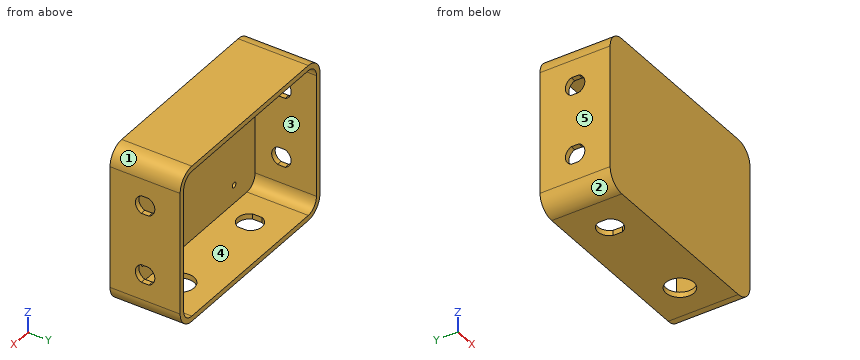
from build123d import *

# Parameters (mm, degrees)
BOSS_EXTRUDE1_DEPTH          = 5
F_3_0_3_DIAMETER_HOLE1_D     = 3
F_3_0_3_DIAMETER_HOLE1_DEPTH = 3
F_3_0_3_DIAMETER_HOLE1_TIP   = 0.901290929
BOSS_EXTRUDE2_DEPTH          = 35
CUT_EXTRUDE1_DEPTH           = 149
CUT_EXTRUDE2_DEPTH           = 35
SKETCH10_R                   = 8
CUT_EXTRUDE3_DEPTH           = 35


with BuildPart() as part:
    # Sketch1 → Boss-Extrude1 (new body)
    with BuildSketch(Plane(origin=(0, 0, 0), x_dir=(1, 0, 0), z_dir=(0, 1, 0))):
        with BuildLine():
            Line((10, 0), (110, 0))
            ThreePointArc((110, 0), (117.071067812, 2.928932188), (120, 10))
            Line((120, 10), (120, 80))
            ThreePointArc((120, 80), (117.071067812, 87.071067812), (110, 90))
            Line((110, 90), (10, 90))
            ThreePointArc((10, 90), (2.928932188, 87.071067812), (0, 80))
            Line((0, 80), (0, 10))
            ThreePointArc((0, 10), (2.928932188, 2.928932188), (10, 0))
        make_face()
    extrude(amount=BOSS_EXTRUDE1_DEPTH)

    # Ø3.0 (3) Diameter Hole1
    with Locations(Plane(origin=(0, 5, 0), x_dir=(1, 0, 0), z_dir=(0, 1, 0))):
        with Locations((99, 76.5), (21, 76.5), (21, 13.5), (99, 13.5)):
            Hole(F_3_0_3_DIAMETER_HOLE1_D / 2, depth=F_3_0_3_DIAMETER_HOLE1_DEPTH)
            with Locations((0, 0, -(F_3_0_3_DIAMETER_HOLE1_DEPTH + F_3_0_3_DIAMETER_HOLE1_TIP / 2))):  # 118° drill point
                Cone(0, F_3_0_3_DIAMETER_HOLE1_D / 2, F_3_0_3_DIAMETER_HOLE1_TIP, mode=Mode.SUBTRACT)

    # Sketch7 → Boss-Extrude2 (add)
    with BuildSketch(Plane(origin=(0, 5, 0), x_dir=(1, 0, 0), z_dir=(0, 1, 0))):
        with BuildLine():
            Line((10, 0), (110, 0))
            ThreePointArc((110, 0), (117.071067812, 2.928932188), (120, 10))
            Line((120, 10), (120, 80))
            ThreePointArc((120, 80), (117.071067812, 87.071067812), (110, 90))
            Line((110, 90), (10, 90))
            ThreePointArc((10, 90), (2.928932188, 87.071067812), (0, 80))
            Line((0, 80), (0, 10))
            ThreePointArc((0, 10), (2.928932188, 2.928932188), (10, 0))
        make_face()
        with BuildLine():
            Line((3, 80), (3, 10))
            ThreePointArc((3, 10), (5.050252532, 5.050252532), (10, 3))
            Line((10, 3), (110, 3))
            ThreePointArc((110, 3), (114.949747468, 5.050252532), (117, 10))
            Line((117, 10), (117, 80))
            ThreePointArc((117, 80), (114.949747468, 84.949747468), (110, 87))
            Line((110, 87), (10, 87))
            ThreePointArc((10, 87), (5.050252532, 84.949747468), (3, 80))
        make_face(mode=Mode.SUBTRACT)
    extrude(amount=BOSS_EXTRUDE2_DEPTH)

    # Sketch8 → Cut-Extrude1 (cut)
    with BuildSketch(Plane.ZY):
        with BuildLine():
            Line((-59.9, 22.189177928), (-59.9, 17.810822072))
            ThreePointArc((-59.9, 17.810822072), (-65, 14.45), (-70.1, 17.810822072))
            Line((-70.1, 17.810822072), (-70.1, 22.189177928))
            ThreePointArc((-70.1, 22.189177928), (-65, 25.55), (-59.9, 22.189177928))
        make_face()
        with BuildLine():
            Line((-19.9, 22.189177928), (-19.9, 17.810822072))
            ThreePointArc((-19.9, 17.810822072), (-25, 14.45), (-30.1, 17.810822072))
            Line((-30.1, 17.810822072), (-30.1, 22.189177928))
            ThreePointArc((-30.1, 22.189177928), (-25, 25.55), (-19.9, 22.189177928))
        make_face()
    extrude(amount=-CUT_EXTRUDE1_DEPTH, mode=Mode.SUBTRACT)

    # Sketch9 → Cut-Extrude2 (cut)
    with BuildSketch(Plane(origin=(0, 0, -90), x_dir=(-1, 0, 0), z_dir=(0, 0, -1))):
        with BuildLine():
            Line((-36.4, 22.709704781), (-36.4, 17.290295219))
            ThreePointArc((-36.4, 17.290295219), (-30, 13.05), (-23.6, 17.290295219))
            Line((-23.6, 17.290295219), (-23.6, 22.709704781))
            ThreePointArc((-23.6, 22.709704781), (-30, 26.95), (-36.4, 22.709704781))
        make_face()
    extrude(amount=-CUT_EXTRUDE2_DEPTH, mode=Mode.SUBTRACT)

    # Sketch10 → Cut-Extrude3 (cut)
    with BuildSketch(Plane(origin=(0, 0, -90), x_dir=(-1, 0, 0), z_dir=(0, 0, -1))):
        with Locations((-90, 20)):
            Circle(SKETCH10_R)
    extrude(amount=-CUT_EXTRUDE3_DEPTH, mode=Mode.SUBTRACT)


solid = part.part
The model under review builds one solid part; all positions refer to its coordinate system, in mm. Face numbers are marked on the shaded views. A direction names the side the tool comes from. Coordinates: 2 decimals unless noted, no trailing zeros. Loops run counter-clockwise (first coordinate to the right, second up) from the corner with the lowest first, then second, coordinate; pieces in that order, holes last.
(1) Consider section A-A, the plane y = 34. Give the boundary of the cut face in (x, z).
Determined:
outline: (0, -80) arc R10 ccw to (10, -90) - (110, -90) arc R10 ccw to (120, -80) - (120, -10) arc R10 ccw to (110, 0) - (10, 0) arc R10 ccw to (0, -10) - close; hole (3, -80) arc R7 ccw to (10, -87) - (110, -87) arc R7 ccw to (117, -80) - (117, -10) arc R7 ccw to (110, -3) - (10, -3) arc R7 ccw to (3, -10) - close
(2) Consider section B-B, the plane x = 90. Give the boundary of the cut face in (y, z).
Determined:
outline: (0, -90) - (12, -90) - (12, -87) - (5, -87) - (5, -3) - (40, -3) - (40, 0) - (0, 0) - close; (28, -90) - (40, -90) - (40, -87) - (28, -87) - close
(3) Consider section D-D, the plane z = -28.5. Give the boundary of the cut face in (x, y).
Determined:
outline: (0, 0) - (120, 0) - (120, 15.69) - (117, 15.69) - (117, 5) - (3, 5) - (3, 15.69) - (0, 15.69) - close; (0, 24.31) - (3, 24.31) - (3, 40) - (0, 40) - close; (117, 24.31) - (120, 24.31) - (120, 40) - (117, 40) - close
(4) Tool access review of the marked faces 4 and 5: name each direction out of +Z, -Z, +X, -X, +Y, -Y from which nothing blocks a thin tool from reaching the whole face with its end or side.
Determined:
face 4: +Y
face 5: +Z, -Z, -X, +Y, -Y
(5) Wall thickness on L1, parallel to X at y = 2.9, z = -76.5; L2, parallel to Z at x = 16.5, y = 29; L3, parallel to X at y = 35.5, z = -55.5: over which ranges is each line inside the solid? List them lowest first.
Determined:
L1: x = 0 to 19.5, 22.5 to 97.5, 100.5 to 120
L2: z = -90 to -87, -3 to 0
L3: x = 0 to 3, 117 to 120
(6) Draft analysis for pull direction X (two halves, no side actions). For the marked faces 1, 2 and 3, state which applies: +X half, -X half, draft (parallel to the pull), parting line (faces both ways), or undercut.
Determined:
face 1: +X half
face 2: -X half
face 3: undercut
(7) Insertion check: P1, Ø0.9, axis at x = 119, y = 19.5, coming from the -Z side; P2, Ø4, axis at x = 19, z = -32.5, coming from the +Y side; P3, Ø1.5, axis at y = 21, z = -88, coming from the -X side. Each pin has a flat end and moves straight along its axis. Give the tip position at first contact, or say it passes through.
Determined:
P1: stops at z = -85.19
P2: stops at y = 5
P3: stops at x = 3.11
(8) Consider section C-C, the plane y = 20. Give the number of separate pieces and of enclosed holes in the cut face, plus the area to 3 significant figures.
Determined:
separate pieces: 6
enclosed holes: 0
area: 971 mm2
